```python
from build123d import *

# Parameters (mm, degrees)
FILLET1_R = 2


with BuildPart() as part:
    # Sketch1 → Revolve1 (revolve)
    with BuildSketch(Plane.YZ, mode=Mode.PRIVATE) as revolve1_sk:
        with BuildLine():
            Line((41.339745962, 12.5), (0, 12.5))
            Line((0, 12.5), (-47.226497308, 12.5))
            ThreePointArc((-47.226497308, 12.5), (-49.726497308, 13.169872981), (-51.556624327, 15))
            Line((-51.556624327, 15), (-52.422649731, 16.5))
            ThreePointArc((-52.422649731, 16.5), (-52.93730682, 17.086805764), (-53.637376906, 17.431935884))
            ThreePointArc((-53.637376906, 17.431935884), (-53.848936639, 17.476488917), (-54.064069414, 17.497945445))
            ThreePointArc((-54.064069414, 17.497945445), (-54.729407093, 17.184079888), (-55, 16.5))
            Line((-55, 16.5), (-55, 7.5))
            Line((-55, 7.5), (55, 7.5))
            Line((55, 7.5), (55, 22.5))
            Line((55, 22.5), (50, 22.5))
            Line((50, 22.5), (45.669872981, 15))
            ThreePointArc((45.669872981, 15), (43.839745962, 13.169872981), (41.339745962, 12.5))
        make_face()
    revolve(revolve1_sk.sketch.rotate(Axis((0, -16.105071473, 0), (0, 1, 0)), 180), axis=Axis((0, -16.105071473, 0), (0, 1, 0)))

    # Fillet1
    fillet1_edges = [part.edges().sort_by_distance(p)[0] for p in [
        (0, 50, 22.5),
    ]]
    fillet(fillet1_edges, radius=FILLET1_R)


solid = part.part
```
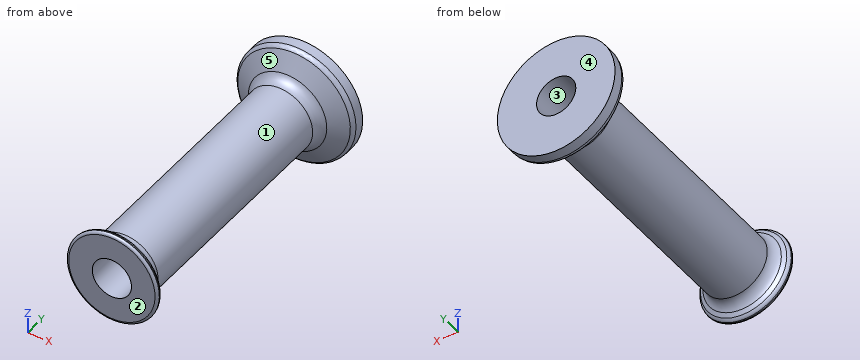
Check sheet for the modelled part. Datum: model origin and axes. Units: mm. Face numbers are marked on the shaded views. A direction names the side the tool comes from. Round coordinates to 2 decimals unless told otherwise and drop trailing zeros. Order: outer loops, then holes, each group sorted by start corner. A loop starts at its lowest first (then second) coordinate and runs counter-clockwise, first axis right, second up. Notation, with made-up numbers: (43.5, 83.5) -> (82.5, 83.5) arc R18 cw to (82.5, 105.5) -> close; hole circle Ø9 at (67, 15.5). An arc over 180 degrees is marked (long way). One line per item, written item: value. Start each with the question number.
Q1. Set-up check for the marked faces 4 and 5: record each of +Z, -Z, +X, -X, +Y, -Y from which the full face is reachable in a straight line by a thin tool's end or side.
Q2. Thickness scan on line 1 (X direction, y = -20.5, z = 0); line 2 (X direction, y = 11.5, z = -10); line 3 (Y direction, x = -8, z = 12). Record the ranges inside material, lowest first.
Q3. Gauge pin test, flat ends, axial feed: pin 1 Ø8 at (y, z) = (-8, 15) entering from -X; pin 2 Ø3 at (y, z) = (-6.5, -1) entering from +X; pin 3 Ø2 at (x, y) = (15, 29.5) entering from +Z; pin 4 Ø3 at (x, y) = (-7, 2.5) entering from +Z (3 decimals). Record the tip position at first contact, or that the pin passes through.
Q4. Mould release check, pull along Y, two halves, no side actions. Record for the marked faces 1, 2 and 3: pulls with the +Y half, pulls with the -Y half, needs draft (parallel to the pull), parting line crosses it, or undercut.
Q5. Cross-section at A-A (y = 11). Record the boundary of the cut face in (x, z), and give its area (3 significant figures).
Completed:
1. face 4: +Z, -Z, +X, -X, +Y
1. face 5: none
2. line 1: x = -12.5 to -7.5, 7.5 to 12.5
2. line 2: x = -7.5 to 7.5
2. line 3: y = -55 to -51.17, 45.28 to 55
3. pin 1: stops at x = -5.94
3. pin 2: stops at x = 12.5
3. pin 3: passes through
3. pin 4: stops at z = 11.225
4. face 1: undercut
4. face 2: pulls with the -Y half
4. face 3: needs draft
5. outline: circle Ø25 at (0, 0); hole circle Ø15 at (0, 0)
5. area: 314 mm²
